Could you check a few things on this model? Use its own coordinates, in mm. Face numbers are marked on the shaded views. Coordinates: 2 decimals unless noted, no trailing zeros. Order: outer loops, then holes, each group sorted by start corner. A loop starts at its lowest first (then second) coordinate and runs counter-clockwise, first axis right, second up. Notation, with made-up numbers: (72, 40) - (97, 40) arc R23 ccw to (97, 51) - close; hole circle Ø11 at (82, 16). An arc over 180 degrees is marked (long way). Answer as a JSON object with one key per item and string values. Group by question number.
(1) Will these pins go through, and if not, where does the flat tip stop? P1, Ø1.5, axis at x = 0, y = -163, coming from the -Z side; P2, Ø1, axis at y = -46, z = 10.5, coming from the -X side; P3, Ø2.5, axis at x = 0, z = -199, coming from the -Y side.
(2) Please list where these lines run through material, in increasing order: probe 1 along Y at (x, z) = (-11, -128); probe 2 along Y at (x, z) = (0.9, -40); probe 3 along Y at (x, z) = (1.1, 40).
(3) Imagine slicing it at B-B, the plane z = -119.5. Write out the boundary of the cut face in (x, y), and give its area (3 significant figures).
(4) Imagine slicing it at C-C, the plane y = -94. Write out the boundary of the cut face in (x, z), and give its area (3 significant figures).
(5) Imagine slicing it at A-A, the plane x = -7.5. Write out the boundary of the cut face in (y, z).
(6) We'd pull the mould along Y, two halves only. Please class the marked faces 1 and 2: pulls with the +Y half, pulls with the -Y half, needs draft (parallel to the pull), parting line crosses it, or undercut.
Autodesk Inventor part; units mm, degrees
ref_plane "YZ Plane" through (0, 0, 0) normal (1, 0, 0) x (0, 1, 0)
ref_plane "XZ Plane" through (0, 0, 0) normal (0, 1, 0) x (-1, 0, 0)
ref_plane "XY Plane" through (0, 0, 0) normal (0, 0, 1) x (1, 0, 0)
sketch "Sketch1" plane through (0, 0, 0) normal (1, 0, 0) x (0, 1, 0)
  line L0 (165, 200) -> (-165, 200)
  line L1 (-165, 200) -> (-165, -200)
  line L2 (-165, -200) -> (165, -200)
  line L3 (165, -200) -> (165, 200)
  line L4 (165, 200) -> (-165, -200) construction
  line L5 (-165, 200) -> (165, -200) construction
  point P0 (0, 0)
  dimension "d0" = 330
  dimension "d1" = 400
extrude "Plate1" add sketch "Sketch1" along normal blind 1.5
sketch "Sketch2" plane through (1.5, 165, 198.5) normal (0, 0, 1) x (1, 0, 0)
  line L0 (0, -330) -> (0, 0)
  line L1 (0, 0) -> (-20, 0)
  line L2 (-20, 0) -> (-20, -330)
  line L3 (-20, -330) -> (0, -330)
edge flange "Flange1" height 20 angle 90 thickness 1.5 bend radius 1.5 thickness toward (0, 0, 1) relief tear relief width 1.5 relief depth 0.75 corner gap 1.5 corner form 2 edges at (0, 0, 200) (0, 165, 0) (0, 0, -200) (0, -165, 0) wall of the first edge with corners at (1.5, -165, 198.5) (1.5, 165, 198.5) (-18.5, 165, 198.5) (-18.5, -165, 198.5)
bend "Bend1"
corner "Corner1"
sketch "Sketch4" plane through (0, 0, 0) normal (-1, 0, 0) x (0, 0, 1)
  circle A0 centre (-40, 11) radius 3.15
  line L0 (0, 0) -> (-5.5711, 0)
  line L1 (0, 0) -> (-6.9523, 0)
  line L2 (0, 0) -> (0, 7.85)
  circle A1 centre (-40, -11) radius 3.15
  circle A2 centre (40, 11) radius 3.15
  circle A3 centre (40, -11) radius 3.15
  dimension "d21" = 6.3
  dimension "d22" = 40
  dimension "d23" = 11
extrude "Cut2" cut sketch "Sketch4" against normal blind 1.5
equation "\"d0\" = C_height"
equation "\"d1\" = C_length"
equation "\"d24\" = Thickness"
equation "\"d2\" = Thickness"
equation "\"d3\" = BendReliefWidth"
equation "\"d4\" = BendReliefDepth"
equation "\"d5\" = MinimumRemnant"
equation "\"d6\" = TransitionRadius"
equation "\"d7\" = C_width"
equation "\"d9\" = BendRadius"
equation "\"d10\" = CornerReliefSize"
equation "\"d11\" = GapSize"
equation "\"d12\" = JacobiRadiusSize"
equation "\"BendRadius\" = Thickness"
equation "\"BendReliefWidth\" = Thickness"
equation "\"BendReliefDepth\" = 0.5 * Thickness"
equation "\"CornerReliefSize\" = 4 * Thickness"
equation "\"MinimumRemnant\" = 2 * Thickness"
equation "\"TransitionRadius\" = BendRadius"
equation "\"JacobiRadiusSize\" = BendRadius"
equation "\"GapSize\" = Thickness"
equation "\"A_width\" = 46"
equation "\"A_joint_diameter\" = 16"
equation "\"A_joint_tolerance\" = 3"
equation "\"l___________\" = 0"
equation "\"l__________\" = 0"
equation "\"C_length\" = 400"
equation "\"C_height\" = 330"
equation "\"l_________\" = 0"
equation "\"rivet_diameter\" = 3.35"
equation "\"plate_thickness\" = 3"
equation "\"l________\" = 0"
equation "\"A_B_spacing\" = 2"
equation "\"L_Piston_Bottom\" = 21"
equation "\"L_Piston_Top\" = 25"
equation "\"thin_plate\" = 1.5"
properties part number "C_plate"
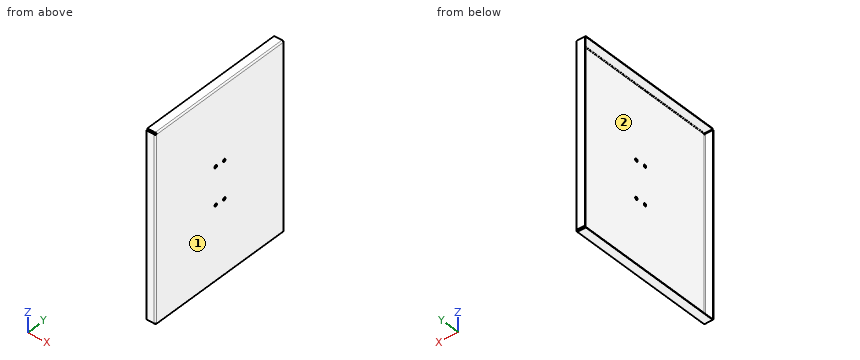
Result set:
{
 "1": {"P1": "stops at z = -197", "P2": "stops at x = 0", "P3": "stops at y = -162"},
 "2": {"probe 1": "y = -165 to -163.5, 163.5 to 165", "probe 2": "y = -163.8 to -14.15, -7.85 to 7.85, 14.15 to 163.8", "probe 3": "y = -163.5 to -14.15, -7.85 to 7.85, 14.15 to 163.5"},
 "3": {"outline": "(-18.5, -165) - (-1.5, -165) arc R3 ccw to (1.5, -162) - (1.5, 162) arc R3 ccw to (-1.5, 165) - (-18.5, 165) - (-18.5, 163.5) - (-1.5, 163.5) arc R1.5 cw to (0, 162) - (0, -162) arc R1.5 cw to (-1.5, -163.5) - (-18.5, -163.5) - close", "area": "548 mm^2"},
 "4": {"outline": "(-18.5, -200) - (-1.5, -200) arc R3 ccw to (1.5, -197) - (1.5, 197) arc R3 ccw to (-1.5, 200) - (-18.5, 200) - (-18.5, 198.5) - (-1.5, 198.5) arc R1.5 cw to (0, 197) - (0, -197) arc R1.5 cw to (-1.5, -198.5) - (-18.5, -198.5) - close", "area": "653 mm^2"},
 "5": {"outline": "(-165, -197.44) - (-163.5, -197.44) - (-163.5, 197.44) - (-165, 197.44) - close; (-162.44, -200) - (162.44, -200) - (162.44, -198.5) - (-162.44, -198.5) - close; (-162.44, 198.5) - (162.44, 198.5) - (162.44, 200) - (-162.44, 200) - close; (163.5, -197.44) - (165, -197.44) - (165, 197.44) - (163.5, 197.44) - close"},
 "6": {"face 1": "needs draft", "face 2": "undercut"}
}
